```python
from build123d import *

# Parameters (mm, degrees)
SALIENTE_EXTRUIR1_DEPTH   = 5
SALIENTE_EXTRUIR1_2_DEPTH = 5
CROQUIS3_W                = 12
CROQUIS3_H                = 12
SALIENTE_EXTRUIR2_DEPTH   = 1.25
CROQUIS4_W                = 12
CROQUIS4_H                = 12
SALIENTE_EXTRUIR3_DEPTH   = 1.25
CROQUIS5_R                = 1.6
CORTAR_EXTRUIR1_DEPTH     = 1.25
CROQUIS9_R                = 1.6
CORTAR_EXTRUIR2_DEPTH     = 1.25
CROQUIS11_W               = 12
CROQUIS11_H               = 12
CROQUIS11_R               = 1.6
SALIENTE_EXTRUIR4_DEPTH   = 24
CROQUIS13_W               = 13
CROQUIS13_H               = 12
SALIENTE_EXTRUIR6_DEPTH   = 30
CROQUIS14_W               = 12
CROQUIS14_H               = 12
SALIENTE_EXTRUIR8_DEPTH   = 18.5
CROQUIS15_W               = 10
CROQUIS15_H               = 5
CORTAR_EXTRUIR3_DEPTH     = 12
CROQUIS16_R               = 1.6
CORTAR_EXTRUIR5_DEPTH     = 32
CROQUIS17_R               = 1.6
CORTAR_EXTRUIR6_DEPTH     = 12


with BuildPart() as part:
    # Croquis2 → Saliente-Extruir1 (new body)
    with BuildSketch(Plane.XY):
        Polygon((-5, -6), (-5, -5), (-5, 5), (-5, 6), (-6, 6), (-6, 5), (-6, -6), align=None)
    extrude(amount=SALIENTE_EXTRUIR1_DEPTH)



with BuildPart() as body_2:
    # Croquis2 → Saliente-Extruir1 2 (new body)
    with BuildSketch(Plane.XY):
        Polygon((5, 5), (5, -5), (5, -6), (6, -6), (6, 6), (5, 6), align=None)
    extrude(amount=SALIENTE_EXTRUIR1_2_DEPTH)


with BuildPart() as part_1:
    add(part.part)

    add(body_2.part)  # Saliente-Extruir2 merges body 2
    # Croquis3 → Saliente-Extruir2 (add)
    with BuildSketch(Plane(origin=(0, 0, 0), x_dir=(-1, 0, 0), z_dir=(0, 0, -1))):
        Rectangle(CROQUIS3_W, CROQUIS3_H)
    extrude(amount=SALIENTE_EXTRUIR2_DEPTH)

    # Croquis4 → Saliente-Extruir3 (add)
    with BuildSketch(Plane.XY.offset(5)):
        Rectangle(CROQUIS4_W, CROQUIS4_H)
    extrude(amount=SALIENTE_EXTRUIR3_DEPTH)

    # Croquis5 → Cortar-Extruir1 (cut)
    with BuildSketch(Plane.XY.offset(6.25)):
        Circle(CROQUIS5_R)
    extrude(amount=-CORTAR_EXTRUIR1_DEPTH, mode=Mode.SUBTRACT)

    # Croquis9 → Cortar-Extruir2 (cut)
    with BuildSketch(Plane.XY):
        Circle(CROQUIS9_R)
    extrude(amount=-CORTAR_EXTRUIR2_DEPTH, mode=Mode.SUBTRACT)

    # Croquis11 → Saliente-Extruir4 (add)
    with BuildSketch(Plane.XY.offset(6.25)):
        Rectangle(CROQUIS11_W, CROQUIS11_H)
        Circle(CROQUIS11_R, mode=Mode.SUBTRACT)
    extrude(amount=SALIENTE_EXTRUIR4_DEPTH)

    # Croquis13 → Saliente-Extruir6 (add)
    with BuildSketch(Plane(origin=(6, 0, 0), x_dir=(0, 0, -1), z_dir=(1, 0, 0))):
        with Locations((-23.75, 0)):
            Rectangle(CROQUIS13_W, CROQUIS13_H)
    extrude(amount=SALIENTE_EXTRUIR6_DEPTH)

    # Croquis14 → Saliente-Extruir8 (add)
    with BuildSketch(Plane(origin=(0, 0, 17.25), x_dir=(-1, 0, 0), z_dir=(0, 0, -1))):
        with Locations((-30, 0)):
            Rectangle(CROQUIS14_W, CROQUIS14_H)
    extrude(amount=SALIENTE_EXTRUIR8_DEPTH)

    # Croquis15 → Cortar-Extruir3 (cut)
    with BuildSketch(Plane(origin=(0, 6, 0), x_dir=(1, 0, 0), z_dir=(0, 1, 0))):
        with Locations((30, -2.5)):
            Rectangle(CROQUIS15_W, CROQUIS15_H)
    extrude(amount=-CORTAR_EXTRUIR3_DEPTH, mode=Mode.SUBTRACT)

    # Croquis16 → Cortar-Extruir5 (cut)
    with BuildSketch(Plane.XY.offset(30.25)):
        Circle(CROQUIS16_R)
        with Locations((30, 0)):
            Circle(CROQUIS16_R)
    extrude(amount=-CORTAR_EXTRUIR5_DEPTH, mode=Mode.SUBTRACT)

    # Croquis17 → Cortar-Extruir6 (cut)
    with BuildSketch(Plane(origin=(0, 6, 0), x_dir=(1, 0, 0), z_dir=(0, 1, 0))):
        with Locations((-3.5, -23.75)):
            Circle(CROQUIS17_R)
        with Locations((33.5, -23.75)):
            Circle(CROQUIS17_R)
    extrude(amount=-CORTAR_EXTRUIR6_DEPTH, mode=Mode.SUBTRACT)


solid = part_1.part
```
Read the model definition and answer for the solid it produces. Units are mm, in the model's axes. A direction names the side the tool comes from. Round coordinates to 2 decimals unless told otherwise and drop trailing zeros. Write each loop counter-clockwise with the first axis right and the second up, starting at its lowest first coordinate (ties: lowest second). Pieces come first, ordered by that corner, then holes. Notation, with made-up numbers: (5.5, -10.75) -> (52.5, -10.75) arc R19 ccw to (52.5, 18.25) -> close; hole circle Ø2 at (81.5, -8.5). An arc over 180 degrees is marked (long way). Answer in a Markdown table with one row per item. Add a question column.
1) Find section A-A, the plane y = 0. State how many separate pieces and enclosed holes the cut face has, and give its area (3 significant figures).
2) Find section D-D, the plane z = 11.5. Determine the outline of the cut face in (x, y), and give its area (3 significant figures).
3) Which of the six approach directions +Z, -Z, +X, -X, +Y, -Y give full straight-line access (tool end or side, diameter ignored) to faces 1 (the face through (31.4, 1.4, -1.25)), 2 (the face through (1.2, 1.4, 0)), 3 (the face through (6, 0, 8))?
4) Determine the mould class of faces 4 (the face through (-3.708, 0.084, 22.164)), 5 (the face through (28.4, 0.07, -0.62)), 6 (the face through (15, 0, 17.25)) for opening direction Z: pulls with the +Z half, pulls with the -Z half, needs draft (parallel to the pull), parting line crosses it, or undercut.
5) Find section C-C, the plane z = 23.75. Determine the outline of the cut face in (x, y).
6) Find section B-B, the plane x = -3.5. Determine the outline of the cut face in (y, z), and give its area (3 significant figures).
7) Consider line 1 (Z direction, x = 33.5, y = 0.75); line 2 (X direction, y = 4.75, z = 2.5); line 3 (X direction, y = -2, z = 23.75). Determine where each line is inside the solid, lowest interval first.
Findings below:
| question | item | result |
|---|---|---|
| 1 | separate pieces | 3 |
| 1 | enclosed holes | 2 |
| 1 | area | 704 mm² |
| 2 | outline | (-6, -6) -> (6, -6) -> (6, 6) -> (-6, 6) -> close; (24, -6) -> (36, -6) -> (36, 6) -> (24, 6) -> close; hole circle Ø3.2 at (0, 0); hole circle Ø3.2 at (30, 0) |
| 2 | area | 272 mm² |
| 3 | face 1 | -Z, +X, -X, +Y, -Y |
| 3 | face 2 | +Y, -Y |
| 3 | face 3 | -Z, +Y, -Y |
| 4 | face 4 | undercut |
| 4 | face 5 | needs draft |
| 4 | face 6 | pulls with the -Z half |
| 5 | outline | (-6, -6) -> (-5.1, -6) -> (-5.1, 6) -> (-6, 6) -> close; (-1.9, -6) -> (31.9, -6) -> (31.9, 6) -> (-1.9, 6) -> close; (35.1, -6) -> (36, -6) -> (36, 6) -> (35.1, 6) -> close; hole circle Ø3.2 at (0, 0); hole circle Ø3.2 at (30, 0) |
| 6 | outline | (-6, -1.25) -> (6, -1.25) -> (6, 0) -> (-6, 0) -> close; (-6, 5) -> (6, 5) -> (6, 22.15) -> (-6, 22.15) -> close; (-6, 25.35) -> (6, 25.35) -> (6, 30.25) -> (-6, 30.25) -> close |
| 6 | area | 280 mm² |
| 7 | line 1 | -1.25 to 0, 5 to 22.15, 25.35 to 30.25 |
| 7 | line 2 | -6 to -5, 5 to 6, 24 to 25, 35 to 36 |
| 7 | line 3 | -6 to -5.1, -1.9 to 31.9, 35.1 to 36 |
